The figure shows three views and two pictorial views of one solid part (mm, origin at its lowest corner). Answer the questions. Give positions to 0.01 mm unless a question says otherwise; leave off trailing zeros. Loops run counter-clockwise (first coordinate to the right, second up) from the corner with the lowest first, then second, coordinate; pieces in that order, holes last. Notation, with made-up numbers: (49, 22.5) - (53, 22.5) arc R22 cw to (53, 42.5) - close; hole circle Ø2 at (26, 47.5). An arc over 180 degrees is marked (long way). Use a Markdown table: item, result. Add a question column.
Item 1: A cutting plane is placed at B-B (x = 85). Determine the outline of the cut face in (y, z).
Item 2: Consider probe 1 along Y at (x, z) = (53, 2.4); probe 2 along X at (y, z) = (35, 1.65). Determine where each line is inside the solid, lowest interval first. Write a range as [from, to].
Item 3: A cutting plane is placed at A-A (z = 2.1). Determine the outline of the cut face in (x, y), plus the area to 3 significant figures.
Item 4: Each of these flat-tipped pins is pushed along its axis until it touches: P1, Ø1.5, axis at y = 1.5, z = 1, coming from the +X side; P2, Ø1.5, axis at x = 126, z = 1, coming from the +Y side; P3, Ø1.5, axis at x = 125.5, z = 1, coming from the -Y side. Where does it stop, or does it pass through?
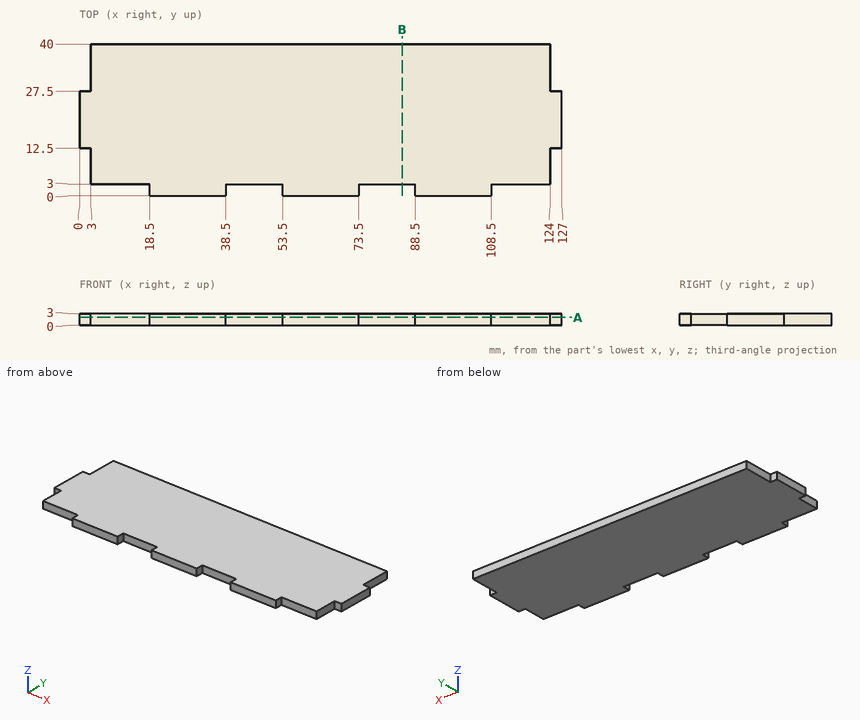
Geometry says:
| question | item | result |
|---|---|---|
| 1 | outline | (3, 0) - (40, 0) - (40, 3) - (3, 3) - close |
| 2 | probe 1 | [3, 40] |
| 2 | probe 2 | [3, 124] |
| 3 | outline | (0, 12.5) - (3, 12.5) - (3, 3) - (18.5, 3) - (18.5, 0) - (38.5, 0) - (38.5, 3) - (53.5, 3) - (53.5, 0) - (73.5, 0) - (73.5, 3) - (88.5, 3) - (88.5, 0) - (108.5, 0) - (108.5, 3) - (124, 3) - (124, 12.5) - (127, 12.5) - (127, 27.5) - (124, 27.5) - (124, 40) - (3, 40) - (3, 27.5) - (0, 27.5) - close |
| 3 | area | 4,750 mm² |
| 4 | P1 | x = 108.5 |
| 4 | P2 | y = 27.5 |
| 4 | P3 | y = 12.5 |
